```python
from build123d import *

# Parameters (mm, degrees)
SKETCH1_W           = 200
SKETCH1_H           = 200
BOSS_EXTRUDE1_DEPTH = 20
SKETCH3_W           = 120
SKETCH3_H           = 120
BOSS_EXTRUDE2_DEPTH = 70
CUT_EXTRUDE1_DEPTH  = 20
SKETCH5_R           = 16
SKETCH5_R_2         = 11
CUT_EXTRUDE2_DEPTH  = 10
FILLET1_R           = 10
FILLET4_R           = 10


with BuildPart() as part:
    # Sketch1 → Boss-Extrude1 (new body)
    with BuildSketch(Plane(origin=(0, 0, 0), x_dir=(1, 0, 0), z_dir=(0, 1, 0))):
        Rectangle(SKETCH1_W, SKETCH1_H)
    extrude(amount=BOSS_EXTRUDE1_DEPTH)

    # Sketch3 → Boss-Extrude2 (add)
    with BuildSketch(Plane.XZ):
        Rectangle(SKETCH3_W, SKETCH3_H)
    extrude(amount=BOSS_EXTRUDE2_DEPTH)

    # Sketch4 → Cut-Extrude1 (cut)
    with BuildSketch(Plane.XZ.offset(70)):
        with BuildLine():
            Line((3.647893136, 28.937904965), (30.991643136, 10.334966059))
            ThreePointArc((30.991643136, 10.334966059), (36.460393136, 0), (30.991643136, -10.334966059))
            Line((30.991643136, -10.334966059), (3.647893136, -28.937904965))
            ThreePointArc((3.647893136, -28.937904965), (-51.039606864, 0), (3.647893136, 28.937904965))
        make_face()
    extrude(amount=-CUT_EXTRUDE1_DEPTH, mode=Mode.SUBTRACT)

    # Sketch5 → Cut-Extrude2 (cut)
    with BuildSketch(Plane.XZ.offset(50)):
        with Locations(Location((-16.039606864, 0, 0), (0, 0, 270))):
            Circle(SKETCH5_R)
        with Locations(Location((23.960393136, 0, 0), (0, 0, 270))):
            Circle(SKETCH5_R_2)
    extrude(amount=-CUT_EXTRUDE2_DEPTH, mode=Mode.SUBTRACT)

    # Fillet1
    fillet1_edges = [part.edges().sort_by_distance(p)[0] for p in [
        (100, 10, 100),
        (-100, 10, 100),
        (-100, 10, -100),
        (100, 10, -100),
    ]]
    fillet(fillet1_edges, radius=FILLET1_R)

    # Fillet4
    fillet4_edges = [part.edges().sort_by_distance(p)[0] for p in [
        (60, 0, 0),
        (0, 0, 60),
        (-60, 0, 0),
        (0, 0, -60),
    ]]
    fillet(fillet4_edges, radius=FILLET4_R)


solid = part.part
```
CAD build for the part. Positions are in the model's coordinates, mm. A direction names the side the tool comes from. Round coordinates to 2 decimals unless told otherwise and drop trailing zeros. Write each loop counter-clockwise with the first axis right and the second up, starting at its lowest first coordinate (ties: lowest second). Pieces come first, ordered by that corner, then holes.
Item 1: Tool access for faces 5 (the flat face through (24, -40, 0)), 6 (the cylindrical face through (0.98, -2.85, -63.01)), 7 (the flat face through (-1, -40, 60)), 8 (the flat face through (60, -40, -1)): list every direction of +Z, -Z, +X, -X, +Y, -Y with a clear straight run to the whole face (end or side of a thin tool).
Filled in:
face 5: -Y
face 6: -Z, +X, -X, -Y
face 7: +Z, +X, -X, -Y
face 8: +Z, -Z, +X, -Y
Item 2: Mould opens along X. For faces 1 (the flat face through (-100, 10, 1)), 2 (the flat face through (-16, -40, 0)), 3 (the cylindrical face through (-51.023, -60.14, -1.062)), 4 (the cylindrical face through (96.99, 10.14, -97.15)) say: released by +X, released by -X, zero draft, split by the parting line, or undercut.
Filled in:
face 1: released by -X
face 2: undercut
face 3: undercut
face 4: released by +X
Item 3: Drill centre lines: L1, parallel to X at y = -46, z = 0; L2, parallel to X at y = -64.25, z = 0; L3, parallel to Y at x = -14, z = 77.5. Where is each one in solid material? Low to high.
Filled in:
L1: x = -60 to -32.04, -0.04 to 12.96, 34.96 to 60
L2: x = -60 to -51.04, 36.46 to 60
L3: y = 0 to 20
Item 4: Drop flat-ended pins along their axis: pin 1 Ø1 at (y, z) = (-4, -16) entering from +X; pin 2 Ø1.5 at (x, y) = (-6.5, -8.5) entering from -Z; pin 3 Ø12 at (x, y) = (-31, -16) entering from +Z. Give the stop position or say it passes through.
Filled in:
pin 1: stops at x = 62.4
pin 2: stops at z = -60.26
pin 3: stops at z = 60
Item 5: Band-saw the part on B-B on z = 0. Write the cut outline in (x, y), then the cut area to 3 significant figures.
Filled in:
outline: (-100, 0) - (-70, 0) arc R10 cw to (-60, -10) - (-60, -70) - (-51.04, -70) - (-51.04, -50) - (-32.04, -50) - (-32.04, -40) - (-0.04, -40) - (-0.04, -50) - (12.96, -50) - (12.96, -40) - (34.96, -40) - (34.96, -50) - (36.46, -50) - (36.46, -70) - (60, -70) - (60, -10) arc R10 cw to (70, 0) - (100, 0) - (100, 20) - (-100, 20) - close
area: 10,200 mm2
Item 6: Band-saw the part on A-A on x = 44.5. Write the cut outline in (y, z), then the cut area to 3 significant figures.
Filled in:
outline: (-70, -60) - (-10, -60) arc R10 cw to (0, -70) - (0, -100) - (20, -100) - (20, 100) - (0, 100) - (0, 70) arc R10 cw to (-10, 60) - (-70, 60) - close
area: 12,400 mm2
Item 7: Band-saw the part on D-D on z = -50.5. Write the cut outline in (x, y).
Filled in:
outline: (-100, 0) - (-70, 0) arc R10 cw to (-60, -10) - (-60, -70) - (60, -70) - (60, -10) arc R10 cw to (70, 0) - (100, 0) - (100, 20) - (-100, 20) - close
Item 8: Band-saw the part on C-C on y = -28. Write the cut outline in (x, z), then the cut area to 3 significant figures.
Filled in:
outline: (-60, -60) - (60, -60) - (60, 60) - (-60, 60) - close
area: 14,400 mm2
